The listing builds one solid part. Answer for the finished solid, in the listing's coordinates (mm). Face numbers are marked on the shaded views. Give positions to 0.01 mm unless a question says otherwise; leave off trailing zeros. Order: outer loops, then holes, each group sorted by start corner. A loop starts at its lowest first (then second) coordinate and runs counter-clockwise, first axis right, second up. Notation, with made-up numbers: (27, 46) -> (67, 46) arc R23 cw to (67, 83) -> close; hole circle Ø5 at (-19, -37). An arc over 180 degrees is marked (long way). Answer as a JSON object with one key per item and string values. Group by question number.
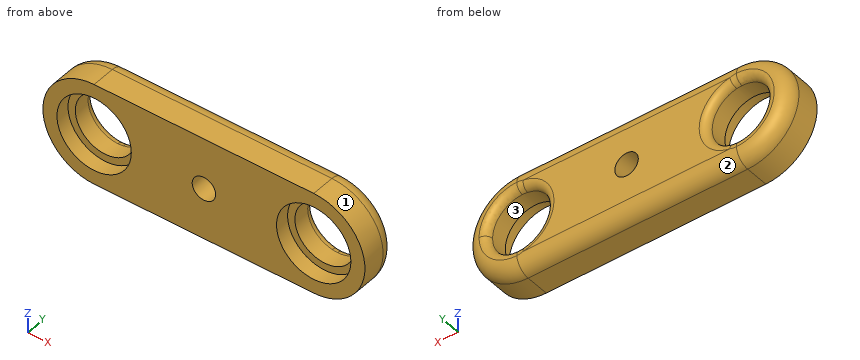
```python
from build123d import *

# Parameters (mm, degrees)
SKETCH1_R           = 4.08
BOSS_EXTRUDE1_DEPTH = 5.2
SKETCH2_R           = 1.6
CUT_EXTRUDE1_DEPTH  = 5.2
SKETCH3_R           = 5.08
CUT_EXTRUDE2_DEPTH  = 1.95
FILLET1_R           = 2
FILLET2_R           = 1


with BuildPart() as part:
    # Sketch1 → Boss-Extrude1 (new body)
    with BuildSketch(Plane(origin=(0, 0, 0), x_dir=(1, 0, 0), z_dir=(0, 1, 0))):
        with BuildLine():
            Line((-15, 7), (15, 7))
            ThreePointArc((15, 7), (22, 0), (15, -7))
            Line((15, -7), (-15, -7))
            ThreePointArc((-15, -7), (-22, 0), (-15, 7))
        make_face()
        with Locations((-15, 0)):
            Circle(SKETCH1_R, mode=Mode.SUBTRACT)
        with Locations((15, 0)):
            Circle(SKETCH1_R, mode=Mode.SUBTRACT)
    extrude(amount=BOSS_EXTRUDE1_DEPTH)

    # Sketch2 → Cut-Extrude1 (cut)
    with BuildSketch(Plane(origin=(0, 5.2, 0), x_dir=(1, 0, 0), z_dir=(0, 1, 0))):
        Circle(SKETCH2_R)
    extrude(amount=-CUT_EXTRUDE1_DEPTH, mode=Mode.SUBTRACT)

    # Sketch3 → Cut-Extrude2 (cut)
    with BuildSketch(Plane.XZ):
        with Locations((-15, 0)):
            Circle(SKETCH3_R)
        with Locations((15, 0)):
            Circle(SKETCH3_R)
    extrude(amount=-CUT_EXTRUDE2_DEPTH, mode=Mode.SUBTRACT)

    # Fillet1
    fillet1_edges = [part.edges().sort_by_distance(p)[0] for p in [
        (22, 5.2, 0),
        (0, 5.2, -7),
        (-22, 5.2, 0),
        (0, 5.2, 7),
    ]]
    fillet(fillet1_edges, radius=FILLET1_R)

    # Fillet2
    fillet2_edges = [part.edges().sort_by_distance(p)[0] for p in [
        (10.92, 5.2, 0),
        (-19.08, 5.2, 0),
    ]]
    fillet(fillet2_edges, radius=FILLET2_R)


solid = part.part
```
(1) A cutting plane is placed at D-D (z = 2.25). State how many separate pieces and enclosed holes the cut face has, and give its area (3 significant figures).
(2) A cutting plane is placed at A-A (x = 0). Determine the outline of the cut face in (y, z), and give its area (3 significant figures).
(3) Find the intervals of material crossed by line 1 along Z through (x, y) = (0, 1.2); line 2 along X through (y, z) = (4.35, 2.25); line 3 along X through (y, z) = (0.35, 0.75), in increasing order. Write a range as [from, to].
(4) A flat-ended cylindrical pin translates along its axis: pin 1 Ø5 at (x, z) = (-14, 0.5) entering from -Y. Find the tip coordinate at first contact, or state that the pin passes through.
(5) For a pull along X with two mould halves and no side action, classify the marked faces 1, 2 and 3 as +X half, -X half, draft (parallel to the pull), parting line (faces both ways), or undercut.
(6) A cutting plane is placed at B-B (y = 2.75). Determine the outline of the cut face in (x, z), and give its area (3 significant figures).
(7) A cutting plane is placed at C-C (x = -6.5). Determine the outline of the cut face in (y, z), and give its area (3 significant figures).
Check sheet entries:
{
 "1": {"separate pieces": "3", "enclosed holes": "0", "area": "142 mm2"},
 "2": {"outline": "(0, -7) -> (3.2, -7) arc R2 ccw to (5.2, -5) -> (5.2, -1.6) -> (0, -1.6) -> close; (0, 1.6) -> (5.2, 1.6) -> (5.2, 5) arc R2 ccw to (3.2, 7) -> (0, 7) -> close", "area": "54.4 mm2"},
 "3": {"line 1": "z = [-7, -1.6], [1.6, 7]", "line 2": "x = [-21.24, -18.42], [-11.58, 11.58], [18.42, 21.24]", "line 3": "x = [-21.96, -20.02], [-9.98, -1.41], [1.41, 9.98], [20.02, 21.96]"},
 "4": {"pin 1": "passes through"},
 "5": {"face 1": "+X half", "face 2": "draft", "face 3": "undercut"},
 "6": {"outline": "(-15, -7) -> (15, -7) arc R7 ccw to (15, 7) -> (-15, 7) arc R7 ccw to start; hole circle Ø8.16 at (-15, 0); hole circle Ø3.2 at (0, 0); hole circle Ø8.16 at (15, 0)", "area": "461 mm2"},
 "7": {"outline": "(0, -7) -> (3.2, -7) arc R2 ccw to (5.2, -5) -> (5.2, 5) arc R2 ccw to (3.2, 7) -> (0, 7) -> close", "area": "71.1 mm2"}
}
